Autodesk Inventor part; units mm, degrees
ref_plane "YZ Plane" through (0, 0, 0) normal (1, 0, 0) x (0, 1, 0)
ref_plane "XZ Plane" through (0, 0, 0) normal (0, 1, 0) x (-1, 0, 0)
ref_plane "XY Plane" through (0, 0, 0) normal (0, 0, 1) x (1, 0, 0)
sketch "Sketch1" plane through (0, 0, 0) normal (0, 0, 1) x (1, 0, 0)
  line L0 (-15.875, 0) -> (15.875, 0)
  line L1 (15.875, 0) -> (15.875, 38.1)
  line L2 (15.875, 38.1) -> (-15.875, 38.1)
  line L3 (-15.875, 38.1) -> (-15.875, 0)
  point P0 (0, 0)
  dimension "d2" = 31.75
  dimension "d3" = 38.1
  dimension "d4" = 15.875
  dimension "d5" = 0
extrude "Extrusion1" add sketch "Sketch1" along normal blind 139.7
sketch "Sketch2" plane through (0, 0, 139.7) normal (0, 0, 1) x (1, 0, 0)
  arc A0 (-12.065, 19.05) -> (12.065, 19.05) centre (0, 19.05) ccw
  line L0 (-15.875, 0) -> (15.875, 0)
  line L1 (12.065, 19.05) -> (12.065, 38.1)
  line L2 (15.875, 38.1) -> (-15.875, 38.1)
  line L3 (-12.065, 19.05) -> (-12.065, 38.1)
  point P0 (0, 0)
  dimension "d8" = 19.05
  dimension "d9" = 24.13
extrude "Extrusion2" cut sketch "Sketch2" against normal through all
sketch "Sketch3" plane through (-15.875, 0, 0) normal (0, -1, 0) x (1, 0, 0)
  circle A0 centre (28.575, 8.89) radius 2
  circle A1 centre (3.175, 130.81) radius 2
  line L0 (15.875, 0) -> (15.875, 139.7) construction
  line L1 (0, 139.7) -> (31.75, 139.7) construction
  line L2 (0, 0) -> (31.75, 0) construction
  line L3 (31.75, 139.7) -> (0, 139.7) construction
  dimension "d12" = 4
  dimension "d13" = 4
  dimension "d14" = 12.7
  dimension "d15" = 8.89
  dimension "d16" = 12.7
  dimension "d17" = 8.89
extrude "Heat Set Inserts" cut sketch "Sketch3" against normal blind 7
sketch "Sketch4" plane through (0, 0, 139.7) normal (0, 0, 1) x (1, 0, 0)
  line L0 (-15.875, 0) -> (15.875, 0)
  line L1 (15.875, 0) -> (15.875, 38.1)
  line L2 (-15.875, 0) -> (15.875, 0)
  line L3 (15.875, 0) -> (15.875, 19.05)
  line L4 (15.875, 19.05) -> (-15.875, 19.05)
  line L5 (-15.875, 19.05) -> (-15.875, 0)
  point P0 (0, 0)
  dimension "d20" = 19.05
extrude "Back Wall" add sketch "Sketch4" along normal blind 1.5875
sketch "Sketch5" plane through (0, 0, 0) normal (0, 0, -1) x (-1, 0, 0)
  line L0 (15.875, 0) -> (-15.875, 0)
  line L1 (15.875, 19.05) -> (15.875, 0)
  line L2 (-15.875, 0) -> (15.875, 0)
  line L3 (15.875, 0) -> (15.875, 10.16)
  line L4 (15.875, 10.16) -> (-15.875, 10.16)
  line L5 (-15.875, 10.16) -> (-15.875, 0)
  point P0 (0, 0)
  dimension "d23" = 10.16
extrude "Extrusion5" add sketch "Sketch5" along normal blind 1.5875
equation "\"d12\" = m3_heat_set_insert"
equation "\"d13\" = m3_heat_set_insert"
equation "\"d18\" = m3_heat_set_depth"
equation "\"m3_heat_set_insert\" = 4"
equation "\"m3_clearance\" = 3.4"
equation "\"m3_heat_set_depth\" = 7"
equation "\"robot_diameter\" = 354"
equation "\"hardboard_thickness\" = 5"
properties part number "NiMH_Holder"
Design review of the part built by this model. Coordinates are the model's own, in mm. A direction names the side the tool comes from. Coordinates: 2 decimals unless noted, no trailing zeros. Order: outer loops, then holes, each group sorted by start corner. A loop starts at its lowest first (then second) coordinate and runs counter-clockwise, first axis right, second up.
1) Clearance check with flat-ended pins moving along their axes: pin 1 (2 mm diameter, centred on x = 12.5, z = 9, fed in from -Y); pin 2 (10 mm diameter, centred on x = 5, y = 27.5, fed in from +Z); pin 3 (12 mm diameter, centred on x = -0.5, z = 46.5, fed in from +Y); pin 4 (6 mm diameter, centred on x = -12.5, y = 28.5, fed in from -Z). State where each tip first meets the part, or that it passes through.
2) Take a section at A-A, the plane z = 8.89. Give the boundary of the cut face in (x, y) (3 decimals).
3) Take a section at B-B, the plane x = 6.5. Give the boundary of the cut face in (y, z), and give its area (3 significant figures).
4) Take a section at C-C, the plane y = 17. Give the boundary of the cut face in (x, z) (1 decimal).
5) Mouldability with a two-part tool opening along X and no side actions: class faces 1 (the flat face through (15.875, 19, 71)), 2 (the flat face through (12.065, 28, 71)), 3 (the flat face through (14, 24, 0)) as +X half, -X half, draft (parallel to the pull), parting line (faces both ways), or undercut.
6) For faces 4 (the cylindrical face through (-11.777, 3.451, 129.036)), 5 (the flat face through (-14, 29, 139.7)), 6 (the flat face through (0, 14, 139.7)), list the 3-axis set-ups (+Z, -Z, +X, -X, +Y, -Y) from which the entire face can be reached by the end or side of a thin tool; tool diameter is ignored.
7) Wall thickness on line 1 along X through (y, z) = (34.5, 58.5) (3 decimals); line 2 along Z through (x, y) = (4.5, 10); line 3 along X through (y, z) = (3, 130.81) (3 decimals): over which ranges is each line inside the solid? List them lowest first.
Returned:
1. pin 1: stops at y = 7
1. pin 2: passes through
1. pin 3: stops at y = 8.89
1. pin 4: stops at z = 0
2. outline: (-15.875, 0) - (10.7, 0) - (10.7, 7) - (14.7, 7) - (14.7, 0) - (15.875, 0) - (15.875, 38.1) - (12.065, 38.1) - (12.065, 19.05) arc R12.065 cw to (-12.065, 19.05) - (-12.065, 38.1) - (-15.875, 38.1) - close
3. outline: (0, -1.59) - (10.16, -1.59) - (10.16, 0) - (8.89, 0) - (8.89, 139.7) - (19.05, 139.7) - (19.05, 141.29) - (0, 141.29) - close
3. area: 1,290 mm2
4. outline: (-15.9, 0) - (-11.9, 0) - (-11.9, 139.7) - (11.9, 139.7) - (11.9, 0) - (15.9, 0) - (15.9, 141.3) - (-15.9, 141.3) - close
5. face 1: +X half
5. face 2: undercut
5. face 3: draft
6. face 4: -Y
6. face 5: +Z, +X, -X, +Y
6. face 6: +Y
7. line 1: x = -15.875 to -12.065, 12.065 to 15.875
7. line 2: z = -1.59 to 0, 139.7 to 141.29
7. line 3: x = -15.875 to -14.7, -10.7 to 15.875
